Read the model definition and answer for the solid it produces. Units are mm, in the model's axes. Face numbers are marked on the shaded views. A direction names the side the tool comes from. Coordinates: 2 decimals unless noted, no trailing zeros. Loops run counter-clockwise (first coordinate to the right, second up) from the corner with the lowest first, then second, coordinate; pieces in that order, holes last. Notation, with made-up numbers: (0, 66) - (46, 66) arc R7 cw to (46, 72) - close; hole circle Ø2 at (9.25, 83.25). An arc over 180 degrees is marked (long way). Use CSV: the item, a comma, the result in double quotes.
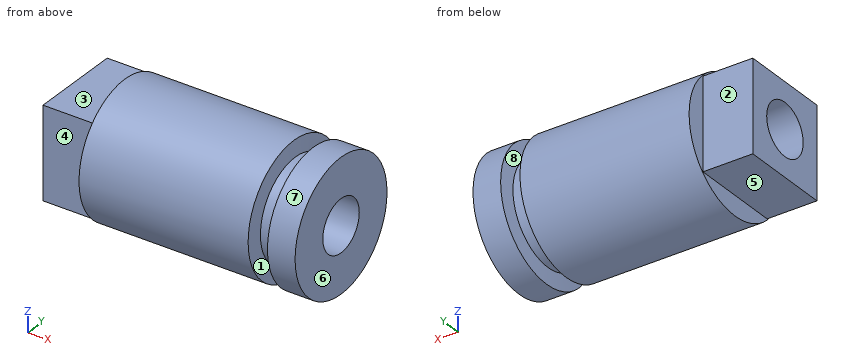
```python
from build123d import *

# Parameters (mm, degrees)
F2_W     = 17.4498
F2_H     = 17.4498
F3_DEPTH = 9.525
F4_R     = 4.953
F5_DEPTH = 50.8


# Not quite as in the source:
# - a feature names something its author has since deleted; it is built from what else it names


with BuildPart() as f1:
    # F0 (on Front) → F1 (revolve)
    with BuildSketch(Plane.XZ):
        Polygon((-22.0124394905, 12.4968), (-22.0124394905, 7.5298989686), (-22.0124394905, 0), (19.2625605095, 0), (19.2625605095, 3.7935770415), (19.2625605095, 12.4968), (13.9844405095, 12.4968), (13.7253605095, 9.525), (10.5503605095, 9.525), (10.2912805095, 12.4968), align=None)
    revolve(axis=Axis((-1.3749394905, 0, 0), (1, 0, 0)))

    # F2 (on face) → F3 (join)
    with BuildSketch(Plane(origin=(-22.0124394905, 0, 0), x_dir=(0, -1, 0), z_dir=(-1, 0, 0))):
        Rectangle(F2_W, F2_H)
    extrude(amount=F3_DEPTH)

    # F4 (on face) → F5 (cut)
    with BuildSketch(Plane.YZ.offset(19.2625605095)):
        Circle(F4_R)
    extrude(amount=-F5_DEPTH, mode=Mode.SUBTRACT)


solid = f1.part
```
Q1. Given P1, Ø6, axis at x = -20.5, z = 8.5, coming from the -Y side; P2, Ø6, axis at y = 9, z = -5.5, coming from the -X side; P3, Ø3, axis at x = -25.5, y = -2, coming from the +Z side; P4, Ø7.5, axis at x = -27, y = -2, coming from the -Z side, each flat-ended and moving along its own axis, determine where each tip first touches the part or whether it passes through.
Reported:
P1,"stops at y = -11.22"
P2,"stops at x = -31.54"
P3,"stops at z = 8.72"
P4,"stops at z = -8.72"
Q2. The part is cut by section C-C on x = -19. Determine the outline of the cut face in (y, z), and give its area (3 significant figures).
Reported:
outline,"circle Ø24.99 at (0, 0); hole circle Ø9.91 at (0, 0)"
area,"414 mm²"
Q3. For a pull along X with two mould halves and no side action, classify the marked faces 6, 7 and 8 as +X half, -X half, draft (parallel to the pull), parting line (faces both ways), or undercut.
Reported:
face 6,"+X half"
face 7,"draft"
face 8,"undercut"
Q4. A tool of negligible diameter and unlimited length cuts with its end or side. For the marked faces 1, 2, 3, 4 and 5, from which of +Z, -Z, +X, -X, +Y, -Y can it reach the whole face along a straight path? Write none if from no direction.
Reported:
face 1,"none"
face 2,"+Z, -Z, -X, +Y"
face 3,"+Z, -X, +Y, -Y"
face 4,"+Z, -Z, -X, -Y"
face 5,"-Z, -X, +Y, -Y"
Q5. The part is cut by section A-A on z = 0. Determine the outline of the cut face in (x, y) (3 decimals).
Reported:
outline,"(-31.537, -8.725) - (-22.012, -8.725) - (-22.012, -12.497) - (10.291, -12.497) - (10.55, -9.525) - (13.725, -9.525) - (13.984, -12.497) - (19.263, -12.497) - (19.263, -4.953) - (-31.537, -4.953) - close; (-31.537, 4.953) - (19.263, 4.953) - (19.263, 12.497) - (13.984, 12.497) - (13.725, 9.525) - (10.55, 9.525) - (10.291, 12.497) - (-22.012, 12.497) - (-22.012, 8.725) - (-31.537, 8.725) - close"
Q6. Find the intervals of material crossed by probe 1 along Z at (x, y) = (0, 0); probe 2 along X at (y, z) = (1, 10.25); probe 3 along Z at (x, y) = (4, -4), in increasing order. Write a range as [from, to].
Reported:
probe 1,"z = [-12.5, -4.95], [4.95, 12.5]"
probe 2,"x = [-22.01, 10.48], [13.79, 19.26]"
probe 3,"z = [-11.84, -2.92], [2.92, 11.84]"
